from build123d import *

# Parameters (mm, degrees)
F1_DEPTH = 20
F2_R     = 15
F3_DEPTH = 25


with BuildPart() as f1:
    # F0 (on Top) → F1 (new body)
    with BuildSketch(Plane.XY):
        with BuildLine():
            Line((66.0472436046, -26.2565443359), (-2.0937833608, 144.0460289628))
            ThreePointArc((-2.0937833608, 144.0460289628), (-26.8847617752, 166.8857654042), (-51.8857822677, 144.2761403347))
            Line((-51.8857822677, 144.2761403347), (-128.0604405721, -26.0728991835))
            ThreePointArc((-128.0604405721, -26.0728991835), (-127.6915622894, -30.833770725), (-123.4960085584, -33.1139676273))
            Line((-123.4960085584, -33.1139676273), (61.4050481416, -33.1139676273))
            ThreePointArc((61.4050481416, -33.1139676273), (65.5455261609, -30.9169021202), (66.0472436046, -26.2565443359))
        make_face()
        with BuildLine():
            Line((-36.2713433227, -23.1139676273), (-108.0700619725, -23.1139676273))
            ThreePointArc((-108.0700619725, -23.1139676273), (-112.2656157035, -20.833770725), (-112.6344939862, -16.0728991835))
            Line((-112.6344939862, -16.0728991835), (-80.009586342, 56.8860323727))
            Line((-80.009586342, 56.8860323727), (-75.9274494544, 66.0148964001))
            Line((-75.9274494544, 66.0148964001), (-42.0002968609, 141.8860323727))
            ThreePointArc((-42.0002968609, 141.8860323727), (-37.6068985787, 152.4926340905), (-27.0002968609, 156.8860323727))
            ThreePointArc((-27.0002968609, 156.8860323727), (-16.3936951431, 152.4926340905), (-12.0002968609, 141.8860323727))
            Line((-12.0002968609, 141.8860323727), (18.2948376146, 66.1704232987))
            Line((18.2948376146, 66.1704232987), (22.0096841973, 56.8860323727))
            Line((22.0096841973, 56.8860323727), (51.2753035904, -16.2565443359))
            ThreePointArc((51.2753035904, -16.2565443359), (50.7735861467, -20.9169021202), (46.6331081274, -23.1139676273))
            Line((46.6331081274, -23.1139676273), (-16.2713433227, -23.1139676273))
            Line((-16.2713433227, -23.1139676273), (-36.2713433227, -23.1139676273))
        make_face(mode=Mode.SUBTRACT)
        Polygon((-80.009586342, 56.8860323727), (-36.2713433227, -23.1139676273), (-16.2713433227, -23.1139676273), (22.0096841973, 56.8860323727), (18.2948376146, 66.1704232987), (-75.9274494544, 66.0148964001), align=None)
        with BuildLine():
            Line((-62.3322616112, 56.8860323727), (5.5765360215, 56.8860323727))
            ThreePointArc((5.5765360215, 56.8860323727), (9.8288943227, 54.5161367201), (10.0501944434, 49.6530119241))
            Line((10.0501944434, 49.6530119241), (-22.0404632685, -14.6377746762))
            ThreePointArc((-22.0404632685, -14.6377746762), (-26.4008005729, -17.403469895), (-30.8819908215, -14.8382125186))
            Line((-30.8819908215, -14.8382125186), (-66.7001307422, 49.4525740817))
            ThreePointArc((-66.7001307422, 49.4525740817), (-66.6431368968, 54.4190847355), (-62.3322616112, 56.8860323727))
        make_face(mode=Mode.SUBTRACT)
        with BuildLine():
            ThreePointArc((-27.0002968609, 156.8860323727), (-37.6068985787, 152.4926340905), (-42.0002968609, 141.8860323727))
            ThreePointArc((-42.0002968609, 141.8860323727), (-27.0002968609, 126.8860323727), (-12.0002968609, 141.8860323727))
            ThreePointArc((-12.0002968609, 141.8860323727), (-16.3936951431, 152.4926340905), (-27.0002968609, 156.8860323727))
        make_face()
    extrude(amount=F1_DEPTH)

    # F2 (on face) → F3 (join)
    with BuildSketch(Plane.XY.offset(20)):
        with Locations((-27.0002968609, 141.8860323727)):
            Circle(F2_R)
    extrude(amount=F3_DEPTH)


solid = f1.part
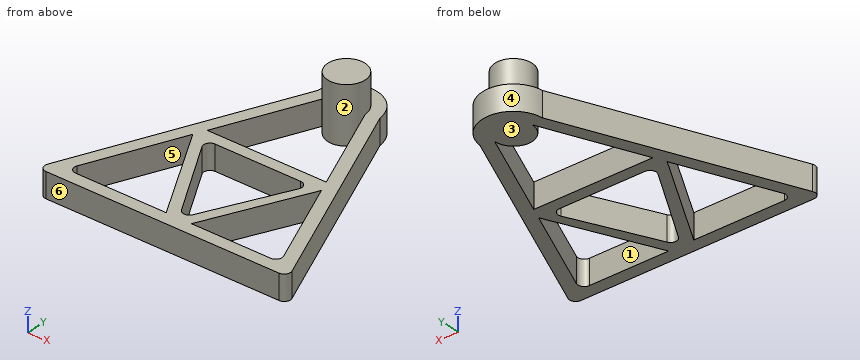
Geometry: final body of the model. Coordinates: model frame, mm. Face numbers are marked on the shaded views. A direction names the side the tool comes from. Round coordinates to 2 decimals unless told otherwise and drop trailing zeros. Write each loop counter-clockwise with the first axis right and the second up, starting at its lowest first coordinate (ties: lowest second). Pieces come first, ordered by that corner, then holes. Notation, with made-up numbers: M -27,84.25 L 2,84.25 A29 cw 2,104.25 Z; hole C 84,86 d8. An arc over 180 degrees is marked long. Write item = value, one per line.
Item 1: Access query for the marked faces 5 and 6. Directions: +Z, -Z, +X, -X, +Y, -Y. A direction counts if a zero-diameter tool reaches every point of the face in a straight line with its end or side. Return the directions, or none.
Findings:
face_5 = +Z, -Z
face_6 = +Z, -Z, +X, -X, -Y
Item 2: Section query C-C on x = -58. Return loops of the section in (y, z), then the cut area to 3 significant figures.
Findings:
outline = M -33.11,0 L -23.11,0 L -23.11,20 L -33.11,20 Z; M 16.63,0 L 33.84,0 L 33.84,20 L 16.63,20 Z; M 56.89,0 L 66.04,0 L 66.04,20 L 56.89,20 Z; M 106.11,0 L 130.6,0 L 130.6,20 L 106.11,20 Z
area = 1,220 mm^2
Item 3: Pin query (flat end, axial travel): P1, Ø10, axis at x = -70, z = 22.5, coming from the -Y side; P2, Ø6, axis at x = -61, z = 7.5, coming from the +Y side; P3, Ø1.5, axis at y = 88, z = 9.5, coming from the -X side; P4, Ø1.5, axis at x = -17.5, z = 10, coming from the +Y side. Return the tip coordinate at first contact, or that it passes through.
Findings:
P1 = -33.11
P2 = 130.6
P3 = -77.39
P4 = 165.3
Item 4: Pull-direction query (X, two-part tool) for the marked faces 1, 2, 3 and 4; classes: pulls with the +X half, pulls with the -X half, needs draft (parallel to the pull), parting line crosses it, or undercut.
Findings:
face_1 = undercut
face_2 = undercut
face_3 = needs draft
face_4 = parting line crosses it
Item 5: Section query A-A on z = 16.5. Return loops of the section in (x, y), then the cut area to 3 significant figures.
Findings:
outline = M -128.06,-26.07 A5 ccw -123.5,-33.11 L 61.41,-33.11 A5 ccw 66.05,-26.26 L -2.09,144.05 A25 ccw -51.89,144.28 Z; hole M -112.63,-16.07 A5 ccw -108.07,-23.11 L -36.27,-23.11 L -80.01,56.89 Z; hole M -75.93,66.01 L 18.29,66.17 L -12,141.89 A15 cw -42,141.89 Z; hole M -66.7,49.45 L -30.88,-14.84 A5 ccw -22.04,-14.64 L 10.05,49.65 A5 ccw 5.58,56.89 L -62.33,56.89 A5 ccw Z; hole M -16.27,-23.11 L 46.63,-23.11 A5 ccw 51.28,-16.26 L 22.01,56.89 Z
area = 9,340 mm^2
Item 6: Section query B-B on y = 109. Return loops of the section in (x, z).
Findings:
outline = M -67.66,0 L -56.71,0 L -56.71,20 L -67.66,20 Z; M 1.16,0 L 11.93,0 L 11.93,20 L 1.16,20 Z
Item 7: Section query D-D on y = 34. Return loops of the section in (x, z), then the cut area to 3 significant figures.
Findings:
outline = M -101.2,0 L -90.24,0 L -90.24,20 L -101.2,20 Z; M -67.5,0 L -58.09,0 L -58.09,20 L -67.5,20 Z; M 2.24,0 L 11.06,0 L 11.06,20 L 2.24,20 Z; M 31.17,0 L 41.94,0 L 41.94,20 L 31.17,20 Z
area = 799 mm^2
Item 8: Material intervals for line 1 along Y through (x, z) = (-21.5, 16) (3 decimals); line 2 along X through (y, z) = (28.5, 18.5); line 3 along Y through (x, z) = (-36, 2), sorted ascending. Write a range as [from, to].
Findings:
line_1 = [-33.114, -13.555], [56.886, 66.105], [127.931, 166.273]
line_2 = [-103.66, -92.7], [-64.49, -55.03], [-0.51, 8.43], [33.37, 44.14]
line_3 = [-33.11, -5.65], [56.89, 66.08], [129.89, 165.21]
